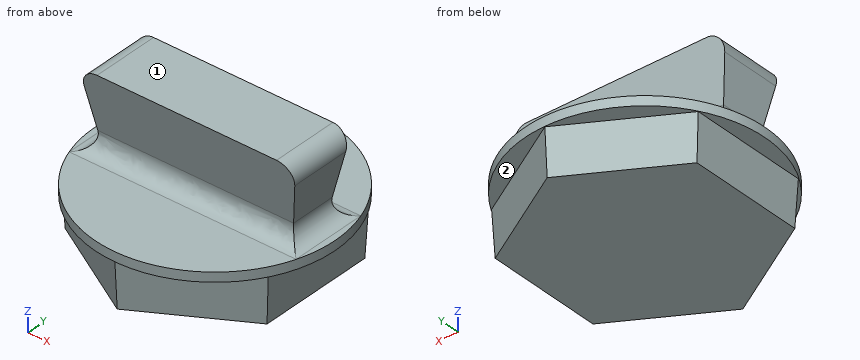
from build123d import *

# Parameters (mm, degrees)
F1_DEPTH = 8.89
F1_TAPER = -3
F2_R     = 19.3087928885
F3_DEPTH = 1.524
F4_W     = 30.48
F4_H     = 6.35
F5_DEPTH = 12.7
F5_TAPER = -10
F6_R     = 2.54


with BuildPart() as f1:
    # F0 (on Top) → F1 (new body)
    with BuildSketch(Plane.XY):
        Polygon((16.256, -9.3854059759), (16.256, 9.3854059759), (0, 18.7708119519), (-16.256, 9.3854059759), (-16.256, -9.3854059759), (0, -18.7708119519), align=None)
    extrude(amount=F1_DEPTH, taper=F1_TAPER)

    # F2 (on face) → F3 (join)
    with BuildSketch(Plane.XY.offset(8.89)):
        Circle(F2_R)
    extrude(amount=-F3_DEPTH)

    # F4 (on face) → F5 (join)
    with BuildSketch(Plane.XY.offset(8.89)):
        Rectangle(F4_W, F4_H)
    extrude(amount=F5_DEPTH, taper=F5_TAPER)

    # F6
    f6_edges = [f1.edges().sort_by_distance(p)[0] for p in [
        (0, 3.175, 8.89),
        (-15.24, 0, 8.89),
        (0, -3.175, 8.89),
        (15.24, 0, 8.89),
        (-17.479353, 0, 21.59),
        (17.479353, 0, 21.59),
    ]]
    fillet(f6_edges, radius=F6_R)


solid = f1.part
Work out the finished part from the listing and answer in its coordinate system (mm). Face numbers are marked on the shaded views. A direction names the side the tool comes from. Round coordinates to 2 decimals unless told otherwise and drop trailing zeros.
1) Given pin 1 Ø1.5 at (y, z) = (-10, 5.5) entering from -X; pin 2 Ø1.5 at (x, y) = (13, 7.5) entering from +Z; pin 3 Ø1 at (x, z) = (-15.5, 7.5) entering from +Y, each flat-ended and moving along its own axis, determine where each tip first touches the part or whether it passes through.
2) A tool of negligible diameter and unlimited length cuts with its end or side. For the marked faces 1 and 2, from which of +Z, -Z, +X, -X, +Y, -Y can it reach the whole face along a straight path? Write none if from no direction.
3) Straight lines are drawn through the part: line 1 (Z direction, x = 4.5, y = 11); line 2 (X direction, y = 14, z = 3.25); line 3 (Y direction, x = 12.5, z = 11). For each, find the intervals that lie inside material, in ascending order.
Completed:
1. pin 1: stops at x = -16.58
1. pin 2: stops at z = 8.89
1. pin 3: stops at y = 12.16
2. face 1: +Z, +X, -X, +Y, -Y
2. face 2: -Z
3. line 1: z = 0 to 8.89
3. line 2: x = -8.6 to 8.6
3. line 3: y = -3.7 to 3.7
